```python
from build123d import *

# Parameters (mm, degrees)
SKETCH_W     = 41
SKETCH_H     = 65
PAD_DEPTH    = 23
SKETCH001_R  = 1.464693
POCKET_DEPTH = 20
FILLET_R     = 2


with BuildPart() as part:
    # Sketch → Pad (new body)
    with BuildSketch(Plane.XY):
        Rectangle(SKETCH_W, SKETCH_H)
    extrude(amount=PAD_DEPTH)

    # Sketch001 → Pocket (cut)
    with BuildSketch(Plane.XY.offset(23)):
        with Locations((17, 29.5)):
            Circle(SKETCH001_R)
        with Locations((-17, 29.5)):
            Circle(SKETCH001_R)
        with Locations((17, -29.5)):
            Circle(SKETCH001_R)
        with Locations((-17, -29.5)):
            Circle(SKETCH001_R)
        Polygon((-12, 30.5), (12, 30.5), (15.75, 25.5), (15.75, -25.5), (13, -32.5), (-13, -32.5), (-15.75, -25.5), (-15.75, 25.5), align=None)
    extrude(amount=-POCKET_DEPTH, mode=Mode.SUBTRACT)

    # Fillet
    fillet_edges = [part.edges().sort_by_distance(p)[0] for p in [
        (-20.5, -32.5, 11.5),
        (0, -32.5, 0),
        (20.5, -32.5, 11.5),
        (20.5, 0, 0),
        (20.5, 32.5, 11.5),
        (0, 32.5, 0),
        (-20.5, 32.5, 11.5),
        (-20.5, 0, 0),
    ]]
    fillet(fillet_edges, radius=FILLET_R)


solid = part.part
```
Part model, mm, in its own coordinate system. A direction names the side the tool comes from. Round coordinates to 2 decimals unless told otherwise and drop trailing zeros. Order: outer loops, then holes, each group sorted by start corner. A loop starts at its lowest first (then second) coordinate and runs counter-clockwise, first axis right, second up. Notation, with made-up numbers: M -5.75,77 L 50.25,77 A24 cw 50.25,98 Z; hole C -15.75,54.5 d10. An arc over 180 degrees is marked long. Put each result on its own line as item: value. Start each with the question number.
1. Slice it at B-B on y = 29.5. List the corners of the cut face in (x, z), then the cut area to 3 significant figures.
2. Drill centre lines: probe 1 along Y at (x, z) = (17, 7); probe 2 along X at (y, z) = (-8.5, 9.5); probe 3 along Y at (x, z) = (-7, 18.25). Where is each one in solid material? Low to high. Write a range as [from, to].
3. Drop flat-ended pins along their axis: pin 1 (9.5 mm diameter, centred on x = 5.5, y = -10.5, fed in from +Z); pin 2 (3 mm diameter, centred on x = -17, y = -29.5, fed in from +Z); pin 3 (10 mm diameter, centred on x = 3.5, z = 17.5, fed in from -Y). Give the stop position or say it passes through.
4. Slice it at C-C on x = -2.5. List the corners of the cut face in (y, z).
5. Tool access for faces 1 (the face through (-20.5, 0, 12)), 2 (the face through (-17, 30, 3)), 3 (the face through (0, 30.5, 13)): list every direction of +Z, -Z, +X, -X, +Y, -Y with a clear straight run to the whole face (end or side of a thin tool).
6. Slice it at D-D on y = 13. List the corners of the cut face in (x, z).
7. Two-plate mould, pull along Y, no slides. Class faces 4 (the face through (-15.75, 0, 13)), 5 (the face through (20.5, 0, 12)), 6 (the face through (0.26, 31.93, 0.6)): +Y half, -Y half, draft (parallel to the pull), parting line (faces both ways), or undercut.
8. Slice it at A-A on z = 14.25. List the corners of the cut face in (x, y), then the cut area to 3 significant figures.
Findings:
1. outline: M -20.5,2 A2 ccw -18.5,0 L 18.5,0 A2 ccw 20.5,2 L 20.5,23 L 18.46,23 L 18.46,3 L 15.54,3 L 15.54,23 L 12.75,23 L 12.75,3 L -12.75,3 L -12.75,23 L -15.54,23 L -15.54,3 L -18.46,3 L -18.46,23 L -20.5,23 Z
1. area: 314 mm2
2. probe 1: [-32.5, -30.96], [-28.04, 28.04], [30.96, 32.5]
2. probe 2: [-20.5, -15.75], [15.75, 20.5]
2. probe 3: [30.5, 32.5]
3. pin 1: z = 3
3. pin 2: z = 23
3. pin 3: y = 30.5
4. outline: M -32.5,2 A2 ccw -30.5,0 L 30.5,0 A2 ccw 32.5,2 L 32.5,23 L 30.5,23 L 30.5,3 L -32.5,3 Z
5. face 1: +Z, -Z, -X, +Y, -Y
5. face 2: +Z
5. face 3: +Z, -Y
6. outline: M -20.5,2 A2 ccw -18.5,0 L 18.5,0 A2 ccw 20.5,2 L 20.5,23 L 15.75,23 L 15.75,3 L -15.75,3 L -15.75,23 L -20.5,23 Z
7. face 4: undercut
7. face 5: draft
7. face 6: +Y half
8. outline: M -20.5,-30.5 A2 ccw -18.5,-32.5 L -13,-32.5 L -15.75,-25.5 L -15.75,25.5 L -12,30.5 L 12,30.5 L 15.75,25.5 L 15.75,-25.5 L 13,-32.5 L 18.5,-32.5 A2 ccw 20.5,-30.5 L 20.5,30.5 A2 ccw 18.5,32.5 L -18.5,32.5 A2 ccw -20.5,30.5 Z; hole C -17,-29.5 d2.93; hole C -17,29.5 d2.93; hole C 17,-29.5 d2.93; hole C 17,29.5 d2.93
8. area: 688 mm2
